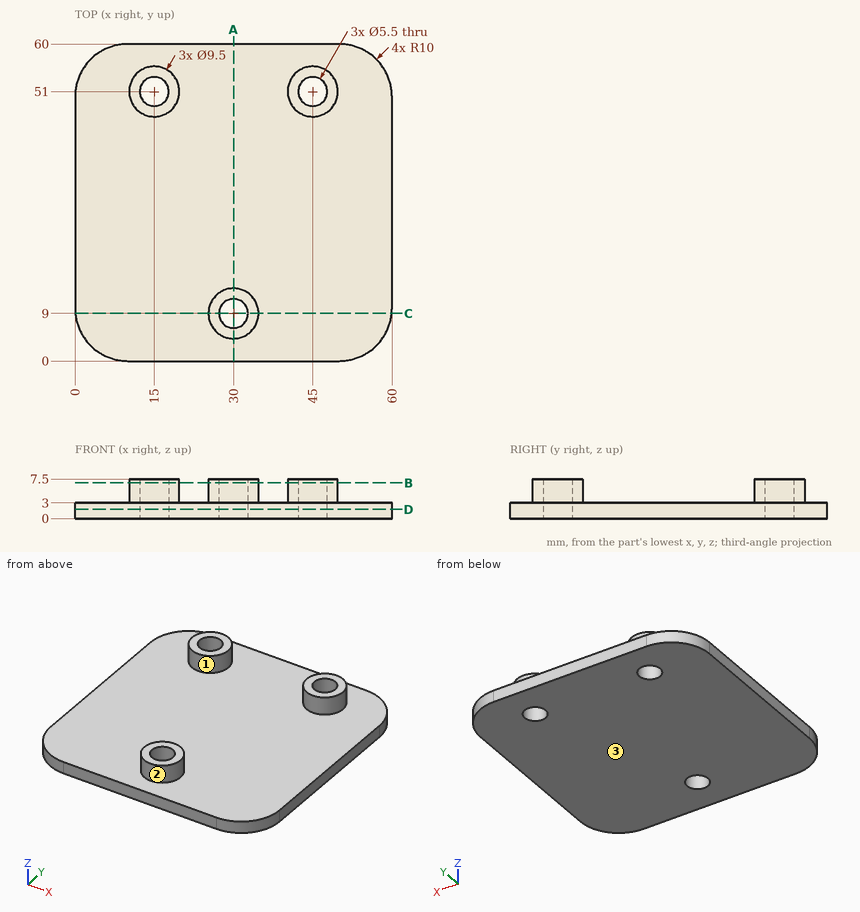
Study the drawing (mm; zero at the part's minimum x, y, z) and answer. Round coordinates to 2 decimals unless told otherwise and drop trailing zeros. Write each loop counter-clockwise with the first axis right and the second up, starting at its lowest first coordinate (ties: lowest second). Pieces come first, ordered by that corner, then holes. Notation, with made-up numbers: (-6, -2) - (6, -2) arc R27 ccw to (6, 32) - close; hole circle Ø7 at (77, 65.5). An arc over 180 degrees is marked (long way). Return JSON: item names as keys, results as strings. Group by question number.
Q1. The part is cut by section B-B on z = 6.75. Write down the section's boundary in (x, y), then the cut area to 3 significant figures.
Q2. The part is cut by section A-A on x = 30. Write down the section's boundary in (y, z).
Q3. The part is cut by section C-C on y = 9. Write down the section's boundary in (x, z), then the cut area to 3 significant figures.
Q4. The part is cut by section D-D on z = 1.75. Write down the section's boundary in (x, y).
Q5. Find the intervals of material crossed by L1, parallel to Y at x = 15, z = 4.5; L2, parallel to Y at x = 30, z = 2.5; L3, parallel to X at y = 49, z = 4.5, in increasing order.
Q6. This flat-tipped pin is pushed along its axis until it touches: pin 1 Ø10 at (x, y) = (39, 32.5) entering from +Z. Where does it stop, or does it pass through?
Q7. The mould has two halves that part along X. Classify the marked faces 1, 2 and 3: released by +X, released by -X, zero draft, split by the parting line, or undercut.
Solved:
{
 "1": {"outline": "circle Ø9.5 at (15, 51); circle Ø9.5 at (30, 9); circle Ø9.5 at (45, 51); hole circle Ø5.5 at (15, 51); hole circle Ø5.5 at (30, 9); hole circle Ø5.5 at (45, 51)", "area": "141 mm²"},
 "2": {"outline": "(0, 0) - (6.25, 0) - (6.25, 7.5) - (4.25, 7.5) - (4.25, 3) - (0, 3) - close; (11.75, 0) - (60, 0) - (60, 3) - (13.75, 3) - (13.75, 7.5) - (11.75, 7.5) - close"},
 "3": {"outline": "(0.05, 0) - (27.25, 0) - (27.25, 7.5) - (25.25, 7.5) - (25.25, 3) - (0.05, 3) - close; (32.75, 0) - (59.95, 0) - (59.95, 3) - (34.75, 3) - (34.75, 7.5) - (32.75, 7.5) - close", "area": "181 mm²"},
 "4": {"outline": "(0, 10) arc R10 ccw to (10, 0) - (50, 0) arc R10 ccw to (60, 10) - (60, 50) arc R10 ccw to (50, 60) - (10, 60) arc R10 ccw to (0, 50) - close; hole circle Ø5.5 at (15, 51); hole circle Ø5.5 at (30, 9); hole circle Ø5.5 at (45, 51)"},
 "5": {"L1": "46.25 to 48.25, 53.75 to 55.75", "L2": "0 to 6.25, 11.75 to 60", "L3": "10.69 to 13.11, 16.89 to 19.31, 40.69 to 43.11, 46.89 to 49.31"},
 "6": {"pin 1": "z = 3"},
 "7": {"face 1": "undercut", "face 2": "split by the parting line", "face 3": "zero draft"}
}
